```python
from build123d import *

# Parameters (mm, degrees)
SKETCH1_R             = 5.075
SKETCH1_R_2           = 1.6
SKETCH1_R_3           = 1.25
SKETCH1_R_4           = 2.1
SKETCH1_R_5           = 0.8
BOSS_EXTRUDE1_DEPTH   = 3.18
CHAMFER1_SIZE         = 2.5
CHAMFER1_SIZE2        = 4.998920521
FILLET2_R             = 3
CHAMFER2_SIZE         = 1.8
FILLET4_R             = 0.5
FILLET7_R             = 0.2
M3X0_5_TAPPED_HOLE1_D = 2.5
M2_TAPPED_HOLE1_D     = 1.6
FILLET8_R             = 0.3
CUT_EXTRUDE5_DEPTH    = 4


with BuildPart() as part:
    # Sketch1 → Boss-Extrude1 (new body)
    with BuildSketch(Plane(origin=(0, 0, 0), x_dir=(0, 0, -1), z_dir=(1, 0, 0))):
        Polygon((0, 0), (0, 30.275), (2, 32.275), (2, 61.31), (22, 61.31), (22, 41.31), (23.8, 41.31), (23.8, 26.21), (15.9, 26.21), (15.9, 15.26), (13.9, 15.26), (13.9, 13.26), (13.4, 13.26), (13.4, 11.86), (25.25, 11.86), (25.25, 6.86), (13.4, 6.86), (13.4, 0), align=None)
        with Locations(Location((7.075, 25.2, 0), (0, 0, 180))):
            Circle(SKETCH1_R, mode=Mode.SUBTRACT)
        with Locations(Location((7, 56.81, 0), (0, 0, 180))):
            Circle(SKETCH1_R_2, mode=Mode.SUBTRACT)
        with Locations(Location((17, 54.81, 0), (0, 0, 180))):
            Circle(SKETCH1_R_2, mode=Mode.SUBTRACT)
        with Locations(Location((22.4, 9.36, 0), (0, 0, 180))):
            Circle(SKETCH1_R_3, mode=Mode.SUBTRACT)
        with Locations(Location((16.4, 9.36, 0), (0, 0, 180))):
            Circle(SKETCH1_R_3, mode=Mode.SUBTRACT)
        with Locations(Location((3.15, 3.95, 0), (0, 0, 180))):
            Circle(SKETCH1_R_4, mode=Mode.SUBTRACT)
        with Locations(Location((3.15, 9.95, 0), (0, 0, 180))):
            Circle(SKETCH1_R_4, mode=Mode.SUBTRACT)
        with Locations(Location((10.15, 2.95, 0), (0, 0, 180))):
            Circle(SKETCH1_R_5, mode=Mode.SUBTRACT)
        with Locations(Location((3.15, 14.95, 0), (0, 0, 180))):
            Circle(SKETCH1_R_5, mode=Mode.SUBTRACT)
    extrude(amount=BOSS_EXTRUDE1_DEPTH)

    # Chamfer1
    chamfer1_edges = [part.edges().sort_by_distance(p)[0] for p in [
        (1.59, 0, -13.4),
    ]]
    chamfer1_side = [part.faces().sort_by_distance(p)[0] for p in [
        (1.59, 0, -6.7),
    ]]
    chamfer(chamfer1_edges, length=CHAMFER1_SIZE, length2=CHAMFER1_SIZE2, reference=chamfer1_side[0])

    # Fillet2
    fillet2_edges = [part.edges().sort_by_distance(p)[0] for p in [
        (1.59, 30.275, 0),
        (1.59, 32.275, -2),
    ]]
    fillet(fillet2_edges, radius=FILLET2_R)

    # Chamfer2
    chamfer2_edges = [part.edges().sort_by_distance(p)[0] for p in [
        (1.59, 61.31, -22),
        (1.59, 61.31, -2),
        (1.59, 41.31, -23.8),
    ]]
    chamfer(chamfer2_edges, length=CHAMFER2_SIZE - 0.0001)  # a hair under: the kernel refuses the full size

    # Fillet4
    fillet4_edges = [part.edges().sort_by_distance(p)[0] for p in [
        (1.59, 39.5101, -23.8),
        (1.59, 59.5101, -22),
        (1.59, 59.5101, -2),
        (1.59, 0, 0),
        (1.59, 4.998920521, -13.4),
    ]]
    fillet(fillet4_edges, radius=FILLET4_R)

    # Fillet7
    fillet7_edges = [part.edges().sort_by_distance(p)[0] for p in [
        (1.59, 13.26, -13.9),
        (1.59, 13.26, -13.4),
    ]]
    fillet(fillet7_edges, radius=FILLET7_R)

    # M3x0.5 Tapped Hole1 (through all)
    with Locations(Plane(origin=(3.18, 0, 0), x_dir=(0, 0, -1), z_dir=(1, 0, 0))):
        with Locations((16.4, 9.36), (22.4, 9.36)):
            Hole(M3X0_5_TAPPED_HOLE1_D / 2)

    # M2 Tapped Hole1 (through all)
    with Locations(Plane(origin=(0, 14.95, -3.15), x_dir=(0, 0, -1), z_dir=(-1, 0, 0))):
        with Locations((0, 0), (7, 12)):
            Hole(M2_TAPPED_HOLE1_D / 2)

    # Fillet8
    fillet8_edges = [part.edges().sort_by_distance(p)[0] for p in [
        (1.59, 15.26, -15.9),
        (1.59, 15.26, -13.9),
    ]]
    fillet(fillet8_edges, radius=FILLET8_R)

    # Sketch13 → Cut-Extrude5 (cut)
    with BuildSketch(Plane(origin=(3.18, 0, 0), x_dir=(0, 0, -1), z_dir=(1, 0, 0))):
        with BuildLine():
            Line((2, 43.846624835), (2, 38.846624835))
            Line((2, 38.846624835), (3.336170487, 38.846624835))
            ThreePointArc((3.336170487, 38.846624835), (19.049907791, 41.271469968), (3.360102459, 43.846624835))
            Line((3.360102459, 43.846624835), (2, 43.846624835))
        make_face()
    extrude(amount=-CUT_EXTRUDE5_DEPTH, mode=Mode.SUBTRACT)


solid = part.part
```
Check sheet for the modelled part. Datum: model origin and axes. Units: mm. A direction names the side the tool comes from. Give positions to 0.01 mm unless a question says otherwise; leave off trailing zeros. Order: outer loops, then holes, each group sorted by start corner. A loop starts at its lowest first (then second) coordinate and runs counter-clockwise, first axis right, second up. Notation, with made-up numbers: M -36,-13.5 L 15,-13.5 A18 cw 15,3.5 Z; hole C 51,43 d9. An arc over 180 degrees is marked long. Answer in a Markdown table with one row per item.
1) Cross-section at B-B, the plane z = -7. Enter the section's corners in (x, y).
Filled sheet:
| item | result |
|---|---|
| outline | M 0,0 L 3.18,0 L 3.18,20.13 L 0,20.13 Z; M 0,30.27 L 3.18,30.27 L 3.18,34.32 L 0,34.32 Z; M 0,48.3 L 3.18,48.3 L 3.18,55.21 L 0,55.21 Z; M 0,58.41 L 3.18,58.41 L 3.18,61.31 L 0,61.31 Z |
2) Gauge pin test, flat ends, axial feed: P1, Ø1, axis at x = 1, y = 36, coming from the +Z side; P2, Ø1, axis at x = 1.5, y = 12.5, coming from the -Z side; P3, Ø1.6, axis at x = 1.5, z = -17, coming from the -Y side. Record the tip position at first contact, or that the pin passes through.
Filled sheet:
| item | result |
|---|---|
| P1 | stops at z = -2 |
| P2 | stops at z = -13.4 |
| P3 | stops at y = 6.86 |
3) Cross-section at C-C, the plane y = 9.36. Enter the section's corners in (x, z), plus the area to 3 significant figures.
Filled sheet:
| item | result |
|---|---|
| outline | M 0,-25.25 L 3.18,-25.25 L 3.18,-23.65 L 0,-23.65 Z; M 0,-21.15 L 3.18,-21.15 L 3.18,-17.65 L 0,-17.65 Z; M 0,-15.15 L 3.18,-15.15 L 3.18,-5.17 L 0,-5.17 Z; M 0,-1.13 L 3.18,-1.13 L 3.18,0 L 0,0 Z |
| area | 51.6 mm2 |
4) Thickness scan on L1, parallel to Z at x = 1.1, y = 25.5; L2, parallel to Y at x = 2.45, z = -16; L3, parallel to Z at x = 0.6, y = 3. Record the ranges inside material, lowest first. Write a range as [from, to].
Filled sheet:
| item | result |
|---|---|
| L1 | z = [-15.9, -12.14], [-2.01, 0] |
| L2 | y = [6.86, 8.18], [10.54, 11.86], [26.21, 35], [47.62, 53.56], [56.06, 61.31] |
| L3 | z = [-12.4, -10.95], [-9.35, -5.02], [-1.28, 0] |
5) Cross-section at D-D, the plane x = 2.2. Count the separate pieces of the cut face and the enclosed holes in it, plus the area to 3 significant figures.
Filled sheet:
| item | result |
|---|---|
| separate pieces | 1 |
| enclosed holes | 9 |
| area | 819 mm2 |
6) Access from +Z, -Z, +X, -X, +Y, -Y to the whole of each face (thin tool, end or side, straight path). Record for faces 1 (the flat face through (2, 0, -6)), 2 (the cylindrical face through (1.57, 9.31, -23.65)), 3 (the flat face through (2, 6.86, -19)), 4 (the flat face through (1.6, 12.5, -13.4)), 5 (the flat face through (2, 50, -22)).
Filled sheet:
| item | result |
|---|---|
| face 1 | +Z, -Z, +X, -X, -Y |
| face 2 | +X, -X |
| face 3 | -Z, +X, -X, -Y |
| face 4 | -Z, +X, -X |
| face 5 | -Z, +X, -X, +Y |
7) Cross-section at A-A, the plane y = 25.2. Enter the section's corners in (x, z), plus the area to 3 significant figures.
Filled sheet:
| item | result |
|---|---|
| outline | M 0,-15.9 L 3.18,-15.9 L 3.18,-12.15 L 0,-12.15 Z; M 0,-2 L 3.18,-2 L 3.18,0 L 0,0 Z |
| area | 18.3 mm2 |
8) Release check for a two-part mould opening along Z. For faces 6 (the flat face through (3.18, 31, -13)), 7 (the cylindrical face through (1.568, 1.868, -3.423)), 8 (the flat face through (2, 51, -2)), 9 (the flat face through (2, 21, -15.9)) record: +Z half, -Z half, draft (parallel to the pull), parting line (faces both ways), or undercut.
Filled sheet:
| item | result |
|---|---|
| face 6 | draft |
| face 7 | undercut |
| face 8 | +Z half |
| face 9 | -Z half |
